Can you work these out from the model? Positions are in its coordinate system, mm. A direction names the side the tool comes from. Give positions to 0.01 mm unless a question says otherwise; leave off trailing zeros. Order: outer loops, then holes, each group sorted by start corner. A loop starts at its lowest first (then second) coordinate and runs counter-clockwise, first axis right, second up. Notation, with made-up numbers: (80.25, 71.5) -> (135.25, 71.5) arc R25 cw to (135.25, 104.5) -> close; hole circle Ø7 at (55.25, -39.75). An arc over 180 degrees is marked (long way). Answer as CSV lines item,"result".
```python
from build123d import *

# Parameters (mm, degrees)
F0_W     = 19.05
F0_H     = 19.05
F1_DEPTH = 57.15
F2_W     = 19.05
F2_H     = 19.05
F3_DEPTH = 19.05
F4_W     = 19.05
F4_H     = 19.05
F5_DEPTH = 19.05


with BuildPart() as f1:
    # F0 (on Top) → F1 (new body)
    with BuildSketch(Plane.XY):
        with Locations((9.525, 9.525)):
            Rectangle(F0_W, F0_H)
    extrude(amount=F1_DEPTH)

    # F2 (on face) → F3 (join)
    with BuildSketch(Plane.YZ.offset(19.05)):
        with Locations((9.525, 28.575)):
            Rectangle(F2_W, F2_H)
    extrude(amount=F3_DEPTH)

    # F4 (on face) → F5 (join)
    with BuildSketch(Plane(origin=(0, 19.05, 0), x_dir=(-1, 0, 0), z_dir=(0, 1, 0))):
        with Locations((-9.525, 28.575)):
            Rectangle(F4_W, F4_H)
    extrude(amount=F5_DEPTH)


solid = f1.part
```
Item 1: For faces 1 (the flat face through (19.05, 9, 9)), 2 (the flat face through (10, 28, 38.1)), 3 (the flat face through (9, 19.05, 9)), 4 (the flat face through (28, 19.05, 28)), which set-ups out of +Z, -Z, +X, -X, +Y, -Y let a thin tool reach every point of the face, with its end or its side?
Numbers:
face 1,"-Z, +X, +Y, -Y"
face 2,"+Z, +X, -X, +Y"
face 3,"-Z, +X, -X, +Y"
face 4,"+Z, -Z, +X, +Y"
Item 2: Imagine slicing it at A-A, the plane x = 4. Please give me the cut outline in (y, z), then the cut area to 3 significant figures.
Numbers:
outline,"(0, 0) -> (19.05, 0) -> (19.05, 19.05) -> (38.1, 19.05) -> (38.1, 38.1) -> (19.05, 38.1) -> (19.05, 57.15) -> (0, 57.15) -> close"
area,"1,450 mm²"
Item 3: Please list where these lines run through material, in increasing order: line 1 along X through (y, z) = (13, 49); line 2 along Z through (x, y) = (11.5, 24).
Numbers:
line 1,"x = 0 to 19.05"
line 2,"z = 19.05 to 38.1"
Item 4: Imagine slicing it at D-D, the plane x = 27. Please give me the cut outline in (y, z), then the cut area to 3 significant figures.
Numbers:
outline,"(0, 19.05) -> (19.05, 19.05) -> (19.05, 38.1) -> (0, 38.1) -> close"
area,"363 mm²"
Item 5: Imagine slicing it at C-C, the plane z = 32. Please give me the cut outline in (x, y), then the cut area to 3 significant figures.
Numbers:
outline,"(0, 0) -> (38.1, 0) -> (38.1, 19.05) -> (19.05, 19.05) -> (19.05, 38.1) -> (0, 38.1) -> close"
area,"1,090 mm²"
Item 6: For pin 1 (5.5 mm diameter, centred on x = 28.5, y = 5, fed in from -Z); pin 2 (9.5 mm diameter, centred on x = 9.5, z = 12, fed in from +Y); pin 3 (10 mm diameter, centred on x = 22.5, y = 33.5, fed in from +Z), each with a flat end and sliding along its axis, tell me the tip position at first contact or that it passes through.
Numbers:
pin 1,"stops at z = 19.05"
pin 2,"stops at y = 19.05"
pin 3,"stops at z = 38.1"
